Read the model definition and answer for the solid it produces. Units are mm, in the model's axes. Face numbers are marked on the shaded views. A direction names the side the tool comes from. Round coordinates to 2 decimals unless told otherwise and drop trailing zeros. Order: outer loops, then holes, each group sorted by start corner. A loop starts at its lowest first (then second) coordinate and runs counter-clockwise, first axis right, second up. Notation, with made-up numbers: M 79.5,-39.5 L 113.5,-39.5 A21 ccw 113.5,-30.5 Z; hole C 66,23 d1. An arc over 180 degrees is marked long. Use one line per item in the form item = value. Start each with the question number.
from build123d import *

# Parameters (mm, degrees)
PAD_DEPTH    = 3
FILLET_R     = 1
CHAMFER_SIZE = 0.4


with BuildPart() as part:
    # Sketch → Pad (new body)
    with BuildSketch(Plane.XY):
        Polygon((4.324051, 21.515991), (4.324051, 27.515991), (12.124051, 27.515991), (12.124051, 21.515991), (18.224051, 21.515991), (18.224051, 16.515991), (-1.775949, 16.515991), (-1.775949, 21.515991), align=None)
    extrude(amount=PAD_DEPTH)

    # Fillet
    fillet_edges = [part.edges().sort_by_distance(p)[0] for p in [
        (18.224051, 21.515991, 1.5),
        (12.124051, 27.515991, 1.5),
        (4.324051, 27.515991, 1.5),
        (18.224051, 16.515991, 1.5),
        (-1.775949, 21.515991, 1.5),
        (-1.775949, 16.515991, 1.5),
    ]]
    fillet(fillet_edges, radius=FILLET_R)

    # Chamfer
    chamfer_edges = [part.edges().sort_by_distance(p)[0] for p in [
        (4.324051, 24.015991, 3),
        (4.616944, 27.223098, 3),
        (1.774051, 21.515991, 3),
        (8.224051, 27.515991, 3),
        (-1.483056, 21.223098, 3),
        (11.831158, 27.223098, 3),
        (-1.775949, 19.015991, 3),
        (12.124051, 24.015991, 3),
        (-1.483056, 16.808884, 3),
        (14.674051, 21.515991, 3),
        (8.224051, 16.515991, 3),
        (17.931158, 21.223098, 3),
        (17.931158, 16.808884, 3),
        (18.224051, 19.015991, 3),
        (4.324051, 24.015991, 0),
        (4.616944, 27.223098, 0),
        (1.774051, 21.515991, 0),
        (8.224051, 27.515991, 0),
        (-1.483056, 21.223098, 0),
        (11.831158, 27.223098, 0),
        (-1.775949, 19.015991, 0),
        (12.124051, 24.015991, 0),
        (-1.483056, 16.808884, 0),
        (14.674051, 21.515991, 0),
        (8.224051, 16.515991, 0),
        (17.931158, 21.223098, 0),
        (17.931158, 16.808884, 0),
        (18.224051, 19.015991, 0),
    ]]
    chamfer(chamfer_edges, length=CHAMFER_SIZE)


solid = part.part
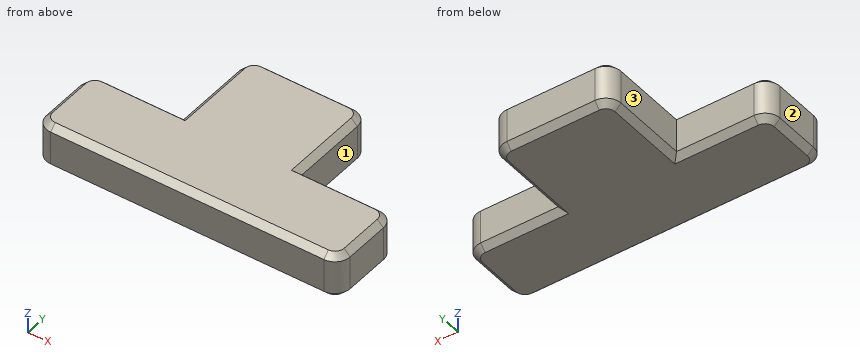
Item 1: Section B-B (y = 23.5) is taken. Write down the section's boundary in (x, z).
Item 2: A tool of negligible diameter and unlimited length cuts with its end or side. For the marked faces 1, 2 and 3, from which of +Z, -Z, +X, -X, +Y, -Y can it reach the whole face along a straight path? Write none if from no direction.
Item 3: Section D-D (z = 0.2) is taken. Write down the section's boundary in (x, y), and give its area (3 significant figures).
Item 4: Given P1, Ø0.7, axis at x = 15.5, z = 1.5, coming from the +Y side; P2, Ø0.7, axis at y = 24, z = 1, coming from the +X side, each flat-ended and moving along its own axis, determine where each tip first touches the part or whether it passes through.
Item 5: Section A-A (z = 1.25) is taken. Write down the section's boundary in (x, y).
Item 6: Find the intervals of material crossed by L1, parallel to Y at x = 17.25, z = 1.9; L2, parallel to X at y = 23.75, z = 2.2; L3, parallel to Y at x = 7, z = 2.85, in increasing order. Write a range as [from, to].
Item 7: Section C-C (x = 0.25) is taken. Write down the section's boundary in (y, z), and give its area (3 significant figures).
The answers:
q1.outline = M 4.32,0.4 L 4.72,0 L 11.72,0 L 12.12,0.4 L 12.12,2.6 L 11.72,3 L 4.72,3 L 4.32,2.6 Z
q2.face_1 = +Z, -Z, +X, +Y
q2.face_2 = +Z, -Z, -X, +Y, -Y
q2.face_3 = +Z, -Z, -X, +Y
q3.outline = M -1.58,17.52 A0.8 ccw -0.78,16.72 L 17.22,16.72 A0.8 ccw 18.02,17.52 L 18.02,20.52 A0.8 ccw 17.22,21.32 L 11.92,21.32 L 11.92,26.52 A0.8 ccw 11.12,27.32 L 5.32,27.32 A0.8 ccw 4.52,26.52 L 4.52,21.32 L -0.78,21.32 A0.8 ccw -1.58,20.52 Z
q3.area = 134 mm²
q4.P1 = 21.52
q4.P2 = 12.12
q5.outline = M -1.78,17.52 A1 ccw -0.78,16.52 L 17.22,16.52 A1 ccw 18.22,17.52 L 18.22,20.52 A1 ccw 17.22,21.52 L 12.12,21.52 L 12.12,26.52 A1 ccw 11.12,27.52 L 5.32,27.52 A1 ccw 4.32,26.52 L 4.32,21.52 L -0.78,21.52 A1 ccw -1.78,20.52 Z
q6.L1 = [16.52, 21.52]
q6.L2 = [4.32, 12.12]
q6.L3 = [16.77, 27.27]
q7.outline = M 16.52,0.4 L 16.92,0 L 21.12,0 L 21.52,0.4 L 21.52,2.6 L 21.12,3 L 16.92,3 L 16.52,2.6 Z
q7.area = 14.7 mm²
